```python
from build123d import *

# Parameters (mm, degrees)
F1_DEPTH = 15
F3_DEPTH = 10.001
F4_W     = 15
F4_H     = 10
F5_DEPTH = 10.001


with BuildPart() as f1:
    # F0 (on Right) → F1 (new body, symmetric)
    with BuildSketch(Plane.YZ):
        Polygon((0, 10), (0, 0), (30, 0), (30, 30), (20, 30), (20, 10), align=None)
    extrude(amount=F1_DEPTH, both=True)

    # F2 (on face) → F3 (cut, through all)
    with BuildSketch(Plane.XZ.offset(-20)):
        Polygon((15, 30), (0, 30), (0, 20), (15, 10), align=None)
    extrude(amount=-F3_DEPTH, mode=Mode.SUBTRACT)

    # F4 (on face) → F5 (cut, through all)
    with BuildSketch(Plane.XY.offset(10)):
        with Locations((7.5, 5)):
            Rectangle(F4_W, F4_H)
    extrude(amount=-F5_DEPTH, mode=Mode.SUBTRACT)


solid = f1.part
```
Geometry check sheet. Reference: the model listing, model coordinates, mm. A direction names the side the tool comes from. Give positions to 0.01 mm unless a question says otherwise; leave off trailing zeros. Order: outer loops, then holes, each group sorted by start corner. A loop starts at its lowest first (then second) coordinate and runs counter-clockwise, first axis right, second up.
1. Access from +Z, -Z, +X, -X, +Y, -Y to the whole of each face (thin tool, end or side, straight path). Record for faces 1 (the face through (0, 5, 5)), 2 (the face through (0, 25, 25)), 3 (the face through (-3, 12, 10)).
2. Section check D-D, the plane z = 14.5. Enter the section's corners in (x, y), and give its area (4 significant figures).
3. Thickness scan on L1, parallel to Y at x = 4, z = 12; L2, parallel to Z at x = 7.75, y = 10.5; L3, parallel to Y at x = 4, z = 1.5. Record the ranges inside material, lowest first.
4. Section check B-B, the plane y = 20.75. Enter the section's corners in (x, z), and give its area (3 significant figures).
5. Section check A-A, the plane x = 3. Enter the section's corners in (y, z), and give its area (3 significant figures).
6. Gauge pin test, flat ends, axial feed: pin 1 Ø12 at (x, y) = (11.5, 23.5) entering from +Z; pin 2 Ø3 at (y, z) = (4, 7.5) entering from +X; pin 3 Ø5 at (x, z) = (5.5, 5.5) entering from -Y. Record the tip position at first contact, or that the pin passes through.
7. Section check C-C, the plane z = 21. Enter the section's corners in (x, y).
Values follow:
1. face 1: +Z, -Z, +X, -Y
1. face 2: +Z, +X, +Y, -Y
1. face 3: +Z, +X, -X, -Y
2. outline: (-15, 20) - (8.25, 20) - (8.25, 30) - (-15, 30) - close
2. area: 232.5 mm2
3. L1: y = 20 to 30
3. L2: z = 0 to 10
3. L3: y = 10 to 30
4. outline: (-15, 0) - (15, 0) - (15, 10) - (0, 20) - (0, 30) - (-15, 30) - close
4. area: 675 mm2
5. outline: (10, 0) - (30, 0) - (30, 18) - (20, 18) - (20, 10) - (10, 10) - close
5. area: 280 mm2
6. pin 1: stops at z = 16.33
6. pin 2: stops at x = 0
6. pin 3: stops at y = 10
7. outline: (-15, 20) - (0, 20) - (0, 30) - (-15, 30) - close
